from build123d import *

# Parameters (mm, degrees)
CHAMFER_2_SIZE        = 0.375
FLATSSKE_W            = 16.5
FLATSSKE_H            = 0.825
FLATS_DEPTH           = 1.975
CLICUTSKE_R           = 0.825
CLINCHINGCUT_DEPTH    = 0.592
CLINCHINGCUTPAT_COUNT = 24
CLINCHINGCUTPAT_ANGLE = 345


with BuildPart() as part:
    # BodySke → Body (revolve)
    with BuildSketch(Plane.XY, mode=Mode.PRIVATE) as body_sk:
        Polygon((5.895636445, 0), (6.335, 0), (6.335, -0.592), (7.2925, -0.592), (7.2925, 0), (8.25, 0), (8.25, 7.9), (4.25, 7.9), (4.25, -1.48), (6.335, -1.48), (6.335, -1.353), (5.895636445, -0.592), align=None)
    revolve(body_sk.sketch.rotate(Axis((0, 0, 0), (0, 1, 0)), 90), axis=Axis((0, 0, 0), (0, 1, 0)))

    # Chamfer 2
    chamfer_2_edges = [part.edges().sort_by_distance(p)[0] for p in [
        (0, 7.9, 8.25),
    ]]
    chamfer(chamfer_2_edges, length=CHAMFER_2_SIZE)

    # FlatsSke → Flats (cut)
    with BuildSketch(Plane(origin=(0, 7.9, 0), x_dir=(-1, 0, 0), z_dir=(0, 1, 0))):
        with Locations((0, 8.25)):
            Rectangle(FLATSSKE_W, FLATSSKE_H)
        with Locations((0, -8.25)):
            Rectangle(FLATSSKE_W, FLATSSKE_H)
    extrude(amount=-FLATS_DEPTH, mode=Mode.SUBTRACT)

    # EndChamferSke → EndChamfer (revolve, cut)
    with BuildSketch(Plane.XY, mode=Mode.PRIVATE) as endchamfer_sk:
        Polygon((5, -1.734), (5, -1.47746), (4.25, -0.952499401), (4.25, -1.734), align=None)
        Polygon((5, 7.9), (4.25, 7.375039401), (4.25, 7.9), align=None)
    revolve(endchamfer_sk.sketch.rotate(Axis((0, -2.54, 0), (0, 1, 0)), 90), axis=Axis((0, -2.54, 0), (0, 1, 0)), mode=Mode.SUBTRACT)

    # CliCutSke → ClinchingCut (cut)
    with BuildSketch(Plane.XZ.offset(0.592)):
        with Locations((0.951862257, 7.230111652)):
            Circle(CLICUTSKE_R)
    clinchingcut = extrude(amount=-CLINCHINGCUT_DEPTH, mode=Mode.SUBTRACT)

    # ClinchingCutPat: ClinchingCut ×24 about axis
    clinchingcutpat_axis = Axis((0, 0, 0), (0, 1, 0))
    for i in range(1, CLINCHINGCUTPAT_COUNT):
        add(clinchingcut.rotate(clinchingcutpat_axis, i * CLINCHINGCUTPAT_ANGLE / (CLINCHINGCUTPAT_COUNT - 1)), mode=Mode.SUBTRACT)


solid = part.part
Source: CAD feature listing. Evaluate the final solid. Frame: model axes, mm. Give positions to 0.01 mm unless a question says otherwise; leave off trailing zeros. Write each loop counter-clockwise with the first axis right and the second up, starting at its lowest first coordinate (ties: lowest second). Pieces come first, ordered by that corner, then holes. Notation, with made-up numbers: (-36.75, -29.75) - (16.25, -29.75) arc R27 ccw to (16.25, 1.25) - close; hole circle Ø5 at (-12.5, 13). An arc over 180 degrees is marked (long way). Write item = value, one per line. Start each with the question number.
Q1. Material intervals for probe 1 along X at (y, z) = (-1.45, 0) (3 decimals); probe 2 along Y at (x, z) = (-3.5, -5); probe 3 along X at (y, z) = (3, 0), sorted ascending.
Q2. Cut plane B-B, the plane y = 3.75. Return loops of the section in (x, z).
Q3. Cut plane A-A, the plane y = 6.75. Return loops of the section in (x, z), then the cut area to 3 significant figures.
Q4. Pin query (flat end, axial travel): pin 1 Ø6 at (x, z) = (1.5, -0.5) entering from +Y; pin 2 Ø4 at (y, z) = (5.5, 5.5) entering from -X; pin 3 Ø0.6 at (x, y) = (1, 6.5) entering from +Z. Return the tip coordinate at first contact, or that it passes through.
Q5. Draft query along X for faces 1 (the cylindrical face through (-4.214, 3.153, 0.553)), 2 (the cylindrical face through (-0.28, -0.3, 6.33)). Return one class per face: +X half, -X half, draft (parallel to the pull), parting line (faces both ways), or undercut.
Computed values:
q1.probe_1 = -6.335 to -4.961, 4.961 to 6.335
q1.probe_2 = -1.48 to -0.95, 0 to 7.9
q1.probe_3 = -8.25 to -4.25, 4.25 to 8.25
q2.outline = circle Ø16.5 at (0, 0); hole circle Ø8.5 at (0, 0)
q3.outline = (-2.58, -7.84) - (2.58, -7.84) arc R8.25 ccw to (2.58, 7.84) - (-2.58, 7.84) arc R8.25 ccw to start; hole circle Ø8.5 at (0, 0)
q3.area = 154 mm²
q4.pin_1 = 7.61
q4.pin_2 = -7.47
q4.pin_3 = 7.84
q5.face_1 = undercut
q5.face_2 = undercut
